The model under review builds one solid part; all positions refer to its coordinate system, in mm. A direction names the side the tool comes from. Round coordinates to 2 decimals unless told otherwise and drop trailing zeros. Write each loop counter-clockwise with the first axis right and the second up, starting at its lowest first coordinate (ties: lowest second). Pieces come first, ordered by that corner, then holes. Notation, with made-up numbers: M 89.25,13.5 L 123.25,13.5 A24 ccw 123.25,38.5 Z; hole C 43.5,50.25 d2. An arc over 180 degrees is marked long. One line per item, written item: value. Start each with the question number.
1) Mouldability with a two-part tool opening along Y and no side actions: class faces 3 (the face through (2, 4, 0)), 4 (the face through (-4, 0, 9)), 5 (the face through (-10.5, 0.1, -6.8)), 6 (the face through (-13.4, -3.43, 6.72)) as +Y half, -Y half, draft (parallel to the pull), parting line (faces both ways), or undercut.
2) Take a section at C-C, the plane x = -8. Write out the cut boundary in (y, z).
3) Tool access review of faces 1 (the face through (-5, 0, -4.5)), 2 (the face through (-14, 0, -7)): name each direction out of +Z, -Z, +X, -X, +Y, -Y from which nothing blocks a thin tool from reaching the whole face with its end or side.
4) Take a section at A-A, the plane y = 0. Write out the cut boundary in (x, z).
5) Take a section at D-D, the plane x = -5. Write out the cut boundary in (y, z).
6) Take a section at B-B, the plane z = 5. Write out the cut boundary in (x, y).
7) Wall thickness on probe 1 along Y at (x, z) = (-8, 6.85); probe 2 along Z at (x, y) = (-0.5, -2.25); probe 3 along Y at (x, z) = (1.5, -2.25): over which ranges is each line inside the solid? List them lowest first.
8) For P1, Ø4, axis at y = 0, z = 0, coming from the -X side, flat-tipped, find the tip position at first contact; note if it passes through.
from build123d import *

# Parameters (mm, degrees)
BOSS_EXTRUDE1_DEPTH     = 4
SKETCH3_R               = 2.5
CUT_EXTRUDE1_DEPTH      = 26.942243542
CUT_EXTRUDE2_DEPTH      = 18.117242769
CUT_EXTRUDE2_DEPTH_BACK = 18.117242769
SKETCH4_R               = 2.5
FILLET1_R               = 2


with BuildPart() as part:
    # Sketch2 → Boss-Extrude1 (new, symmetric)
    with BuildSketch(Plane(origin=(0, 0, 0), x_dir=(1, 0, 0), z_dir=(0, 1, 0))):
        with BuildLine():
            Line((0, 4.5), (-14, 4.5))
            Line((-14, 4.5), (-14, 9))
            Line((-14, 9), (5, 9))
            ThreePointArc((5, 9), (6.464466094, 5.464466094), (10, 4))
            Line((10, 4), (10, -4))
            ThreePointArc((10, -4), (6.464466094, -5.464466094), (5, -9))
            Line((5, -9), (-14, -9))
            Line((-14, -9), (-14, -4.5))
            Line((-14, -4.5), (0, -4.5))
            Line((0, -4.5), (0, 4.5))
        make_face()
    extrude(amount=BOSS_EXTRUDE1_DEPTH, both=True)

    # Sketch3 → Cut-Extrude1 (cut, through all)
    with BuildSketch(Plane(origin=(10, 0, 0), x_dir=(0, 0, -1), z_dir=(1, 0, 0))):
        Circle(SKETCH3_R)
    extrude(amount=-CUT_EXTRUDE1_DEPTH, mode=Mode.SUBTRACT)

    # Sketch4 → Cut-Extrude2 (cut, two sides: drawn at the far end of the back side and taken through both)
    with BuildSketch(Plane.XY.offset(-CUT_EXTRUDE2_DEPTH_BACK)):
        with Locations((-8, 0)):
            Circle(SKETCH4_R)
    extrude(amount=CUT_EXTRUDE2_DEPTH + CUT_EXTRUDE2_DEPTH_BACK, mode=Mode.SUBTRACT)

    # Fillet1
    fillet1_edges = [part.edges().sort_by_distance(p)[0] for p in [
        (-14, -4, -6.75),
        (-14, 4, 6.75),
        (-14, -4, 6.75),
        (-14, 4, -6.75),
    ]]
    fillet(fillet1_edges, radius=FILLET1_R)


solid = part.part
Checked values:
1. face 3: +Y half
1. face 4: draft
1. face 5: undercut
1. face 6: -Y half
2. outline: M -4,-9 L -2.5,-9 L -2.5,-4.5 L -4,-4.5 Z; M -4,4.5 L -2.5,4.5 L -2.5,9 L -4,9 Z; M 2.5,-9 L 4,-9 L 4,-4.5 L 2.5,-4.5 Z; M 2.5,4.5 L 4,4.5 L 4,9 L 2.5,9 Z
3. face 1: -X, +Y, -Y
3. face 2: +Z, -Z, -X, +Y, -Y
4. outline: M -14,-9 L -10.5,-9 L -10.5,-4.5 L -14,-4.5 Z; M -14,4.5 L -10.5,4.5 L -10.5,9 L -14,9 Z; M -5.5,-9 L 5,-9 A5 cw 10,-4 L 10,-2.5 L 0,-2.5 L 0,-4.5 L -5.5,-4.5 Z; M -5.5,4.5 L 0,4.5 L 0,2.5 L 10,2.5 L 10,4 A5 cw 5,9 L -5.5,9 Z
5. outline: M -4,-9 L 4,-9 L 4,-4.5 L -4,-4.5 Z; M -4,4.5 L 4,4.5 L 4,9 L -4,9 Z
6. outline: M -14,-2 A2 ccw -12,-4 L 7,-4 L 7,4 L -12,4 A2 ccw -14,2 Z; hole C -8,0 d5
7. probe 1: y = -4 to -2.5, 2.5 to 4
7. probe 2: z = -9 to -4.5, 4.5 to 9
7. probe 3: y = -4 to -1.09, 1.09 to 4
8. P1: passes through
